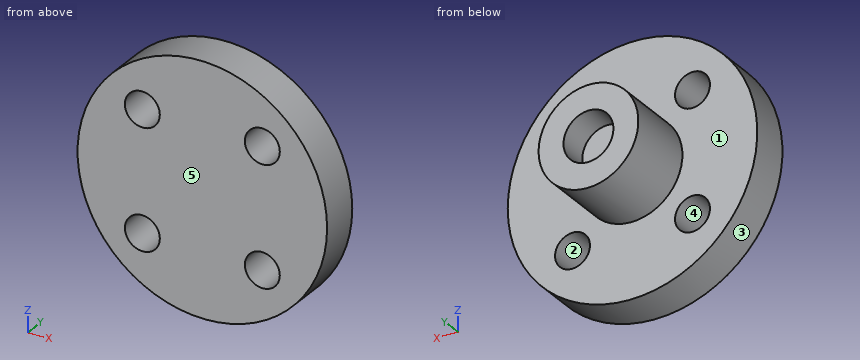
from build123d import *

# Parameters (mm, degrees)
SKETCH1_R           = 12.5
BOSS_EXTRUDE1_DEPTH = 4
SKETCH2_R           = 5
SKETCH2_R_2         = 2.5
BOSS_EXTRUDE2_DEPTH = 7
CUT_EXTRUDE1_REACH  = 6
SKETCH3_R           = 1.75
SKETCH2_2_R         = 2.5
BOSS_EXTRUDE3_DEPTH = 4


with BuildPart() as part:
    # Sketch1 → Boss-Extrude1 (new body)
    with BuildSketch(Plane(origin=(0, 0, 0), x_dir=(1, 0, 0), z_dir=(0, 1, 0))):
        Circle(SKETCH1_R)
    extrude(amount=BOSS_EXTRUDE1_DEPTH)

    # Sketch2 → Boss-Extrude2 (add)
    with BuildSketch(Plane(origin=(0, 4, 0), x_dir=(1, 0, 0), z_dir=(0, 1, 0))):
        Circle(SKETCH2_R)
        Circle(SKETCH2_R_2, mode=Mode.SUBTRACT)
    extrude(amount=BOSS_EXTRUDE2_DEPTH)

    # Sketch3 → Cut-Extrude1 (cut, up to next)
    with BuildSketch(Plane(origin=(0, 4, 0), x_dir=(1, 0, 0), z_dir=(0, 1, 0)), mode=Mode.PRIVATE) as cut_extrude1_sk1:
        with Locations((-6.01040764, 6.01040764)):
            Circle(SKETCH3_R)
    cut_extrude1_tool1 = extrude(cut_extrude1_sk1.sketch, amount=-CUT_EXTRUDE1_REACH, mode=Mode.PRIVATE) & part.part
    add(cut_extrude1_tool1.solids().sort_by_distance((-6.010408, 4, -6.010408))[0], mode=Mode.SUBTRACT)
    # Sketch3 → Cut-Extrude1 (cut, up to next)
    with BuildSketch(Plane(origin=(0, 4, 0), x_dir=(1, 0, 0), z_dir=(0, 1, 0)), mode=Mode.PRIVATE) as cut_extrude1_sk2:
        with Locations((6.01040764, 6.01040764)):
            Circle(SKETCH3_R)
    cut_extrude1_tool2 = extrude(cut_extrude1_sk2.sketch, amount=-CUT_EXTRUDE1_REACH, mode=Mode.PRIVATE) & part.part
    add(cut_extrude1_tool2.solids().sort_by_distance((6.010408, 4, -6.010408))[0], mode=Mode.SUBTRACT)
    # Sketch3 → Cut-Extrude1 (cut, up to next)
    with BuildSketch(Plane(origin=(0, 4, 0), x_dir=(1, 0, 0), z_dir=(0, 1, 0)), mode=Mode.PRIVATE) as cut_extrude1_sk3:
        with Locations((6.01040764, -6.01040764)):
            Circle(SKETCH3_R)
    cut_extrude1_tool3 = extrude(cut_extrude1_sk3.sketch, amount=-CUT_EXTRUDE1_REACH, mode=Mode.PRIVATE) & part.part
    add(cut_extrude1_tool3.solids().sort_by_distance((6.010408, 4, 6.010408))[0], mode=Mode.SUBTRACT)
    # Sketch3 → Cut-Extrude1 (cut, up to next)
    with BuildSketch(Plane(origin=(0, 4, 0), x_dir=(1, 0, 0), z_dir=(0, 1, 0)), mode=Mode.PRIVATE) as cut_extrude1_sk4:
        with Locations((-6.01040764, -6.01040764)):
            Circle(SKETCH3_R)
    cut_extrude1_tool4 = extrude(cut_extrude1_sk4.sketch, amount=-CUT_EXTRUDE1_REACH, mode=Mode.PRIVATE) & part.part
    add(cut_extrude1_tool4.solids().sort_by_distance((-6.010408, 4, 6.010408))[0], mode=Mode.SUBTRACT)

    # Sketch2_2 → Boss-Extrude3 (add)
    with BuildSketch(Plane(origin=(0, 4, 0), x_dir=(1, 0, 0), z_dir=(0, 1, 0))):
        Circle(SKETCH2_2_R)
    extrude(amount=BOSS_EXTRUDE3_DEPTH)


solid = part.part
The model under review builds one solid part; all positions refer to its coordinate system, in mm. Face numbers are marked on the shaded views. A direction names the side the tool comes from. Round coordinates to 2 decimals unless told otherwise and drop trailing zeros. Write each loop counter-clockwise with the first axis right and the second up, starting at its lowest first coordinate (ties: lowest second). Pieces come first, ordered by that corner, then holes. Notation, with made-up numbers: M 53,-16.75 L 66,-16.75 A15 ccw 66,10.25 Z; hole C 28,-30.75 d7. An arc over 180 degrees is marked long. Use a Markdown table: item, result. Add a question column.
Q1. We need section B-B, the plane x = 0. State the section outline as (y, z) points.
Q2. We need section A-A, the plane z = 0. State the section outline as (x, y) points, plus the area to 3 significant figures.
Q3. Machinability: for the marked faces 1 and 2, which of the approach directions +Z, -Z, +X, -X, +Y, -Y give a long, thin tool a straight path to every point of the face, cutting with its end or side? Answer none if there is none.
Q4. To check wall thickness, follow line 1 (X direction, y = 10.25, z = 0); line 2 (Y direction, x = -4.5, z = 8.5). State the ranges of each line that lie inside material, in increasing order.
Q5. Insertion check: pin 1 (4 mm diameter, centred on y = 8, z = 2, fed in from +X); pin 2 (6 mm diameter, centred on y = 3, z = -4, fed in from -X); pin 3 (2.5 mm diameter, centred on x = -0.5, z = 0, fed in from +Y). Each pin has a flat end and moves straight along its axis. Give the tip position at first contact, or say it passes through.
Q6. The part is to be moulded in two halves that separate along Z. For the marked faces 3, 4 and 5, say which applies: pulls with the +Z half, pulls with the -Z half, needs draft (parallel to the pull), parting line crosses it, or undercut.
Q7. We need section D-D, the plane y = 5.25. State the section outline as (x, z) points.
Q8. We need section C-C, the plane y = 2.25. State the section outline as (x, z) points.
Findings below:
| question | item | result |
|---|---|---|
| 1 | outline | M 0,-12.5 L 4,-12.5 L 4,-5 L 11,-5 L 11,-2.5 L 8,-2.5 L 8,2.5 L 11,2.5 L 11,5 L 4,5 L 4,12.5 L 0,12.5 Z |
| 2 | outline | M -12.5,0 L 12.5,0 L 12.5,4 L 5,4 L 5,11 L 2.5,11 L 2.5,8 L -2.5,8 L -2.5,11 L -5,11 L -5,4 L -12.5,4 Z |
| 2 | area | 155 mm² |
| 3 | face 1 | +Y |
| 3 | face 2 | +Y, -Y |
| 4 | line 1 | x = -5 to -2.5, 2.5 to 5 |
| 4 | line 2 | y = 0 to 4 |
| 5 | pin 1 | stops at x = 5 |
| 5 | pin 2 | stops at x = -12.46 |
| 5 | pin 3 | stops at y = 8 |
| 6 | face 3 | parting line crosses it |
| 6 | face 4 | undercut |
| 6 | face 5 | needs draft |
| 7 | outline | C 0,0 d10 |
| 8 | outline | C 0,0 d25; hole C -6.01,-6.01 d3.5; hole C -6.01,6.01 d3.5; hole C 6.01,-6.01 d3.5; hole C 6.01,6.01 d3.5 |
